CAD build for the part. Positions are in the model's coordinates, mm. Coordinates: 2 decimals unless noted, no trailing zeros. Order: outer loops, then holes, each group sorted by start corner. A loop starts at its lowest first (then second) coordinate and runs counter-clockwise, first axis right, second up.
from build123d import *

# Parameters (mm, degrees)
F0_W     = 254
F0_H     = 127
F1_DEPTH = 203.2
F2_SIZE2 = 126.99999
F2_SIZE  = 126.99999


# Not quite as in the source:
# - a fillet or chamfer is up to 0.001 mm smaller than in the source, because OpenCascade refuses the exact size


with BuildPart() as f1:
    # F0 (on Front) → F1 (new body)
    with BuildSketch(Plane.XZ):
        with Locations((-127, 63.5)):
            Rectangle(F0_W, F0_H)
    extrude(amount=F1_DEPTH)

    # F2 (size 127 and 127 in the source; OpenCascade refuses exactly that, so slightly less here)
    f2_edges = [f1.edges().sort_by_distance(p)[0] for p in [
        (0, -101.6, 0),
    ]]
    chamfer(f2_edges, length=F2_SIZE, length2=F2_SIZE2)


solid = f1.part
1) Slice it at B-B (z = 65.5). List the corners of the cut face in (x, y).
2) Drill centre lines: probe 1 along X at (y, z) = (-43, 51.5); probe 2 along X at (y, z) = (-109.5, 105); probe 3 along Z at (x, y) = (-108, -192). Where is each one in solid material? Low to high.
3) Slice it at C-C (x = -18). List the corners of the cut face in (y, z), plus the area to 3 significant figures.
4) Pin check, flat tips, straight feed: P1, Ø1, axis at y = -54, z = 16, coming from the +X side; P2, Ø1, axis at y = -22, z = 66, coming from the +X side. Stop position of each tip, or through.
Worked out:
1. outline: (-254, -203.2) - (-61.5, -203.2) - (-61.5, 0) - (-254, 0) - close
2. probe 1: x = -254 to -75.5
2. probe 2: x = -254 to -22
2. probe 3: z = 19 to 127
3. outline: (-203.2, 109) - (0, 109) - (0, 127) - (-203.2, 127) - close
3. area: 3,660 mm2
4. P1: stops at x = -110.5
4. P2: stops at x = -60.5
